Geometry: final body of the model. Coordinates: model frame, mm. Give positions to 0.01 mm unless a question says otherwise; leave off trailing zeros. Loops run counter-clockwise (first coordinate to the right, second up) from the corner with the lowest first, then second, coordinate; pieces in that order, holes last.
1. Section B-B, the plane y = 4.5. Output: boundary loops of the cut face in (x, z) (3 decimals).
2. Draft query along Z for faces 1 (the face through (-1.71, 3.13, -43.95)), 2 (the face through (6.35, 3, -20)), 3 (the face through (0.14, 3.13, 6.35)), 4 (the face through (0.69, 3.13, 3.1)). Return one class per face: +Z half, -Z half, draft (parallel to the pull), parting line (faces both ways), or undercut.
3. Section C-C, the plane x = 0. Output: boundary loops of the cut face in (y, z) (3 decimals), then the cut area to 3 significant figures.
4. Section A-A, the plane z = -12.7. Output: boundary loops of the cut face in (x, y) (3 decimals), then the cut area to 3 significant figures.
5. Section D-D, the plane z = -42.5. Output: boundary loops of the cut face in (x, y), then the cut area to 3 significant figures.
6. Material intervals for line 1 along Z through (x, y) = (0, 4) (3 decimals); line 2 along Z through (x, y) = (-1.5, 3); line 3 along X through (y, z) = (5, -12.7) (3 decimals), sorted ascending.
Autodesk Inventor part; units mm, degrees
ref_plane "YZ Plane" through (0, 0, 0) normal (1, 0, 0) x (0, 1, 0)
ref_plane "XZ Plane" through (0, 0, 0) normal (0, 1, 0) x (-1, 0, 0)
ref_plane "XY Plane" through (0, 0, 0) normal (0, 0, 1) x (1, 0, 0)
sketch "Sketch1" plane through (0, 0, 0) normal (0, 1, 0) x (-1, 0, 0)
  circle A0 centre (0, 0) radius 3.175
  circle A1 centre (0, -12.7) radius 3.175
  line L0 (-6.35, -15.875) -> (-6.35, 0)
  line L1 (6.35, 0) -> (6.35, -15.875)
  line L2 (-6.35, 0) -> (-3.175, 0)
  line L3 (-6.35, -15.875) -> (-6.35, -41.275)
  circle A2 centre (0, -41.275) radius 3.175
  arc A3 (-6.35, -41.275) -> (6.35, -41.275) centre (0, -41.275) ccw
  line L4 (-6.35, -41.275) -> (-6.35, -15.875)
  line L5 (-6.35, -15.875) -> (0, -15.875)
  line L6 (6.35, -15.875) -> (6.35, -41.275)
  arc A4 (6.35, 0) -> (-6.35, 0) centre (0, 0) ccw
  point P0 (6.35, -7.9375)
  dimension "d0" = 6.35
  dimension "d1" = 6.35
  dimension "d14" = 6.35
  dimension "d17" = 12.7
  dimension "d18" = 6.35
  dimension "d19" = 6.35
  dimension "d20" = 12.7
  dimension "d21" = 12.7
  dimension "d22" = 12.7
extrude "Extrusion1" add sketch "Sketch1" along normal blind 6.35
properties part number "Gear to Finger Connect"
Answers below:
1. outline: (-6.35, -41.275) arc R6.35 ccw to (6.35, -41.275) - (6.35, 0) arc R6.35 ccw to (-6.35, 0) - close; hole circle Ø6.35 at (0, -41.275); hole circle Ø6.35 at (0, -12.7); hole circle Ø6.35 at (0, 0)
2. face 1: undercut
2. face 2: draft
2. face 3: +Z half
2. face 4: undercut
3. outline: (0, -47.625) - (6.35, -47.625) - (6.35, -44.45) - (0, -44.45) - close; (0, -38.1) - (6.35, -38.1) - (6.35, -15.875) - (0, -15.875) - close; (0, -9.525) - (6.35, -9.525) - (6.35, -3.175) - (0, -3.175) - close; (0, 3.175) - (6.35, 3.175) - (6.35, 6.35) - (0, 6.35) - close
3. area: 222 mm2
4. outline: (-6.35, 0) - (-3.175, 0) - (-3.175, 6.35) - (-6.35, 6.35) - close; (3.175, 0) - (6.35, 0) - (6.35, 6.35) - (3.175, 6.35) - close
4. area: 40.3 mm2
5. outline: (-6.23, 0) - (-2.93, 0) - (-2.93, 6.35) - (-6.23, 6.35) - close; (2.93, 0) - (6.23, 0) - (6.23, 6.35) - (2.93, 6.35) - close
5. area: 41.9 mm2
6. line 1: z = -47.625 to -44.45, -38.1 to -15.875, -9.525 to -3.175, 3.175 to 6.35
6. line 2: z = -47.45 to -44.07, -38.48 to -15.5, -9.9 to -2.8, 2.8 to 6.17
6. line 3: x = -6.35 to -3.175, 3.175 to 6.35
